Autodesk Inventor part; units mm, degrees
ref_plane "YZ Plane" through (0, 0, 0) normal (1, 0, 0) x (0, 1, 0)
ref_plane "XZ Plane" through (0, 0, 0) normal (0, 1, 0) x (-1, 0, 0)
ref_plane "XY Plane" through (0, 0, 0) normal (0, 0, 1) x (1, 0, 0)
sketch "Sketch1" plane through (0, 0, 0) normal (0, 0, 1) x (1, 0, 0)
  line L0 (-28.6909, 41.0213) -> (-8.6909, 41.0213)
  line L1 (-8.6909, 41.0213) -> (-8.6909, 1.0213)
  line L2 (-8.6909, 1.0213) -> (-28.6909, 1.0213)
  line L3 (-28.6909, 1.0213) -> (-28.6909, 41.0213)
  circle A0 centre (-24.6909, 37.0213) radius 1.5
  circle A1 centre (-12.6909, 37.0213) radius 1.5
  dimension "d0" = 20
  dimension "d1" = 40
  dimension "d4" = 3
  dimension "d5" = 3
  dimension "d7" = 4
  dimension "d8" = 4
  dimension "d9" = 4
  dimension "d10" = 4
extrude "Extrusion1" add sketch "Sketch1" along normal blind 2
equation "\"d4\" = d5"
equation "\"d7\" = d9"
equation "\"d8\" = d10"
properties part number "Placa PCB 40x20"
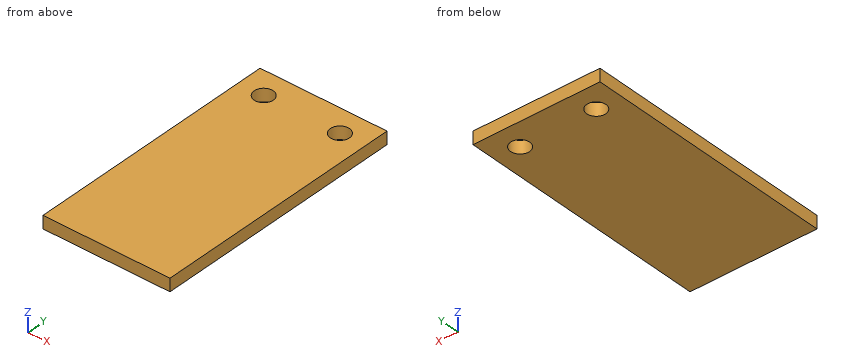
CAD build for the part. Positions are in the model's coordinates, mm. Coordinates: 2 decimals unless noted, no trailing zeros. Loops run counter-clockwise (first coordinate to the right, second up) from the corner with the lowest first, then second, coordinate; pieces in that order, holes last. Notation, with made-up numbers: (75.25, 14.5) - (132.25, 14.5) arc R20 ccw to (132.25, 33.5) - close; hole circle Ø3 at (-24, 26). An arc over 180 degrees is marked (long way). Return JSON: item names as keys, results as strings.
1. Probe L1, parallel to Y at x = -24.75, z = 1.2; L2, parallel to Y at x = -23.5, z = 1.45. List the from-to ranges inside material, lowest first. Write a range as from..to.
Result:
{"L1": "y = 1.02..35.52, 38.52..41.02", "L2": "y = 1.02..36.11, 37.93..41.02"}
2. Band-saw the part on A-A (x = -11.75). Give the cut face in (y, z).
Result:
{"outline": "(1.02, 0) - (35.85, 0) - (35.85, 2) - (1.02, 2) - close; (38.19, 0) - (41.02, 0) - (41.02, 2) - (38.19, 2) - close"}
3. Band-saw the part on B-B (z = 1.3). Give the cut face in (x, y), and give its area (3 significant figures).
Result:
{"outline": "(-28.69, 1.02) - (-8.69, 1.02) - (-8.69, 41.02) - (-28.69, 41.02) - close; hole circle Ø3 at (-24.69, 37.02); hole circle Ø3 at (-12.69, 37.02)", "area": "786 mm2"}
